Design review of the part built by this model. Coordinates are the model's own, in mm. A direction names the side the tool comes from. Round coordinates to 2 decimals unless told otherwise and drop trailing zeros. Order: outer loops, then holes, each group sorted by start corner. A loop starts at its lowest first (then second) coordinate and runs counter-clockwise, first axis right, second up. Notation, with made-up numbers: M 65,-5.75 L 109,-5.75 A24 ccw 109,14.25 Z; hole C 78,47 d5. An arc over 180 degrees is marked long. Write each question's results on one line, items separated by ' | '. Start each with the question number.
Item 1: Take a section at C-C, the plane z = 51.5. Write out the cut boundary in (x, y).
Item 2: Clearance check with flat-ended pins moving along their axes: pin 1 (2.5 mm diameter, centred on x = -1.5, z = 23, fed in from -Y); pin 2 (2.5 mm diameter, centred on x = -0.5, y = -9.5, fed in from +Z); pin 3 (4 mm diameter, centred on y = 15.5, z = 0, fed in from +X). State where each tip first meets the part, or that it passes through.
Item 3: Take a section at A-A, the plane x = 2.75. Write out the cut boundary in (y, z).
Item 4: Take a section at B-B, the plane y = -20. Write out the cut boundary in (x, z), plus the area to 3 significant figures.
Item 5: Machinability: for faces 5 (the flat face through (0, 17.727, 28)), 6 (the flat face through (0.4, -24.823, -3.5)), 7 (the flat face through (0, -1, -9.092)), 8 (the flat face through (0, 18.227, 28)), 9 (the flat face through (-4.525, 20, 12)), which of the approach directions +Z, -Z, +X, -X, +Y, -Y give a long, thin tool a straight path to every point of the face, cutting with its end or side? Answer none if there is none.
Item 6: The part is to be moulded in two halves that separate along Z. For faces 1 (the flat face through (4.025, 19, 12)), 2 (the flat face through (-4.025, 19, 15)), 3 (the flat face through (0, 24.153, 25)), 4 (the flat face through (1, 18, 59.908)), say which applies: +Z half, -Z half, draft (parallel to the pull), parting line (faces both ways), or undercut.
Item 7: Wall thickness on line 1 (Y direction, x = 0.75, z = 37.5); line 2 (Z direction, x = 1.5, y = 8.5); line 3 (Z direction, x = -3.25, y = 20.5): over which ranges is each line inside the solid? List them lowest first. Write a range as [from, to].
```python
from build123d import *

# Parameters (mm, degrees)
SKETCH2_W   = 9.050402016
SKETCH2_H   = 6.425792272
SKETCH2_W_2 = 8.050402016
SKETCH2_H_2 = 5.425792272


with BuildPart() as part:
    # Sweep-Thin1: sweep along a path in Sketch1
    with BuildLine(Plane(origin=(0, 0, 0), x_dir=(0, 0, -1), z_dir=(1, 0, 0))) as sweep_thin1_path:
        Line((-59.908239877, 20.940148661), (6.379118135, 20.940148661))
        Line((6.379118135, 20.940148661), (6.379118135, -24.823090134))
    # Sketch2 → Sweep-Thin1 (sweep)
    with BuildSketch(Plane(origin=(0, 20.940148661, 59.908239877), x_dir=(-1, 0, 0), z_dir=(0, 0, -1))):
        Rectangle(SKETCH2_W, SKETCH2_H)
        Rectangle(SKETCH2_W_2, SKETCH2_H_2, mode=Mode.SUBTRACT)
    sweep(path=sweep_thin1_path.line, transition=Transition.RIGHT)


solid = part.part
```
Results list:
1) outline: M -4.53,17.73 L 4.53,17.73 L 4.53,24.15 L -4.53,24.15 Z; hole M -4.03,18.23 L 4.03,18.23 L 4.03,23.65 L -4.03,23.65 Z
2) pin 1: y = 17.73 | pin 2: z = -3.17 | pin 3: through
3) outline: M -24.82,-9.59 L 24.15,-9.59 L 24.15,59.91 L 23.65,59.91 L 23.65,-9.09 L -24.82,-9.09 Z; M -24.82,-3.67 L 18.23,-3.67 L 18.23,59.91 L 17.73,59.91 L 17.73,-3.17 L -24.82,-3.17 Z
4) outline: M -4.53,-9.59 L 4.53,-9.59 L 4.53,-3.17 L -4.53,-3.17 Z; hole M -4.03,-9.09 L 4.03,-9.09 L 4.03,-3.67 L -4.03,-3.67 Z | area: 14.5 mm²
5) face 5: +Z, +X, -X, -Y | face 6: +Z, -Z, +X, -X, -Y | face 7: -Y | face 8: +Z | face 9: +Z, -Z, -X, +Y, -Y
6) face 1: undercut | face 2: undercut | face 3: draft | face 4: +Z half
7) line 1: [17.73, 18.23], [23.65, 24.15] | line 2: [-9.59, -9.09], [-3.67, -3.17] | line 3: [-9.59, -9.09]
